from build123d import *

# Parameters (mm, degrees)
RESSALTO_EXTRUS_O1_DEPTH             = 52.5
ESBO_O3_W                            = 10
ESBO_O3_H                            = 4
RESSALTO_EXTRUS_O2_DEPTH             = 5
ESBO_O4_R                            = 1.7
ESBO_O4_W                            = 2.5
ESBO_O4_H                            = 5.6
RESSALTO_EXTRUS_O3_DEPTH             = 10
ESBO_O5_R                            = 1.65
CORTE_EXTRUS_O1_DEPTH                = 6
RESSALTO_EXTRUS_O4_REACH             = 12.6
ESBO_O6_W                            = 10
ESBO_O6_H                            = 2
RESSALTO_EXTRUS_O4_DIRECTION_2_REACH = 117.6


with BuildPart() as part:
    # Esboço1 → Ressalto-extrusão1 (new body, symmetric)
    with BuildSketch(Plane.XY):
        Polygon((0, 0), (0, 2), (5, 2), (5, 4), (10, 4), (10, 2), (20, 2), (20, 0), align=None)
    extrude(amount=RESSALTO_EXTRUS_O1_DEPTH, both=True)

    # Esboço3 → Ressalto-extrusão2 (add)
    with BuildSketch(Plane.XY.offset(52.5)):
        with Locations((5, 2)):
            Rectangle(ESBO_O3_W, ESBO_O3_H)
    extrude(amount=-RESSALTO_EXTRUS_O2_DEPTH)

    # Esboço4 → Ressalto-extrusão3 (add, through all)
    with BuildSketch(Plane(origin=(10, 0, 0), x_dir=(0, 0, -1), z_dir=(1, 0, 0))):
        Polygon((-52.5, 9.5), (-63.1, 9.5), (-63.1, 0), (-52.5, 0), (-52.5, 3.742943079), align=None)
        with Locations((-56.7, 4.7)):
            Circle(ESBO_O4_R, mode=Mode.SUBTRACT)
        with Locations((-59.85, 4.7)):
            Rectangle(ESBO_O4_W, ESBO_O4_H, mode=Mode.SUBTRACT)
    ressalto_extrus_o3 = extrude(amount=-RESSALTO_EXTRUS_O3_DEPTH)

    # Esboço5 → Corte-extrusão1 (cut)
    with BuildSketch(Plane.XY.offset(63.1)):
        with Locations((4, 4.7)):
            Circle(ESBO_O5_R)
    corte_extrus_o1 = extrude(amount=-CORTE_EXTRUS_O1_DEPTH, mode=Mode.SUBTRACT)

    # Espelhar1: Ressalto-extrusão3, Corte-extrusão1 across plane
    add(ressalto_extrus_o3.mirror(Plane.XY))
    add(corte_extrus_o1.mirror(Plane.XY), mode=Mode.SUBTRACT)

    # Ressalto-extrusão4: up to this face of the body (flat: up to its plane)
    ressalto_extrus_o4_end = Plane(part.part.faces().sort_by_distance((5, 9.362068858, 63.1))[0])
    # Esboço6 → Ressalto-extrusão4 (add, up to the picked face)
    with BuildSketch(Plane.XY.offset(52.5), mode=Mode.PRIVATE) as ressalto_extrus_o4_sk1:
        with Locations((15, 1)):
            Rectangle(ESBO_O6_W, ESBO_O6_H)
    ressalto_extrus_o4_tool1 = split(extrude(ressalto_extrus_o4_sk1.sketch, amount=RESSALTO_EXTRUS_O4_REACH, mode=Mode.PRIVATE), bisect_by=ressalto_extrus_o4_end, keep=Keep.BOTH, mode=Mode.PRIVATE)
    add(ressalto_extrus_o4_tool1.solids().sort_by_distance((15, 1, 52.5))[0])

    # Ressalto-extrusão4 direction 2: up to this face of the body (flat: up to its plane)
    ressalto_extrus_o4_direction_2_end = Plane(part.part.faces().sort_by_distance((5, 9.362068858, -63.1))[0])
    # Esboço6 → Ressalto-extrusão4 direction 2 (add, up to the picked face)
    with BuildSketch(Plane.XY.offset(52.5), mode=Mode.PRIVATE) as ressalto_extrus_o4_direction_2_sk1:
        with Locations((15, 1)):
            Rectangle(ESBO_O6_W, ESBO_O6_H)
    ressalto_extrus_o4_direction_2_tool1 = split(extrude(ressalto_extrus_o4_direction_2_sk1.sketch, amount=-RESSALTO_EXTRUS_O4_DIRECTION_2_REACH, mode=Mode.PRIVATE), bisect_by=ressalto_extrus_o4_direction_2_end, keep=Keep.BOTH, mode=Mode.PRIVATE)
    add(ressalto_extrus_o4_direction_2_tool1.solids().sort_by_distance((15, 1, 52.5))[0])


solid = part.part
Could you check a few things on this model? Use its own coordinates, in mm. A direction names the side the tool comes from. Give positions to 0.01 mm unless a question says otherwise; leave off trailing zeros. Order: outer loops, then holes, each group sorted by start corner. A loop starts at its lowest first (then second) coordinate and runs counter-clockwise, first axis right, second up.
Item 1: If we section it at A-A, the plane z = 7.5: Write out the boundary of the cut face in (x, y), plus the area to 3 significant figures.
Item 2: I need wall thicknesses on line 1 (X direction, y = 4.7, z = -62.45); line 2 (Y direction, x = 6.75, z = -56.7); line 3 (Z direction, x = 4.25, y = 4.7). Which ranges of each line are inside material? Lowest first, please.
Item 3: I'm going to push flat-ended pins straight in: pin 1 (11 mm diameter, centred on x = 4, z = 14.5, fed in from +Y); pin 2 (0.6 mm diameter, centred on y = 3, z = -9.5, fed in from -X); pin 3 (2 mm diameter, centred on x = 14.5, z = 6.5, fed in from +Y). Where does each tip first touch, or does it pass through?
Item 4: If we section it at B-B, the plane x = 17.5: Write out the boundary of the cut face in (y, z), plus the area to 3 significant figures.
Item 5: For faces 5 (the face through (5, 7, 52.5)), 6 (the face through (5, 3, -2)), 7 (the face through (5, 7.5, -60)), 8 (the face through (3.785, 6.336, 62.114)), which set-ups out of +Z, -Z, +X, -X, +Y, -Y let a thin tool reach every point of the face, with its end or its side?
Item 6: If we section it at C-C, the plane z = 51: Write out the boundary of the cut face in (x, y).
Item 7: If we mould it in two halves opening along X, with no side actions, what happens to faces 1 (the face through (4.89, 6.09, 58.03)), 2 (the face through (5, 9.5, 58)), 3 (the face through (0, 1.6, -0.3)), 4 (the face through (4.89, 6.09, -58.03))? For each: pulls with the +X half, pulls with the -X half, needs draft (parallel to the pull), parting line crosses it, or undercut.
Values:
1. outline: (0, 0) - (20, 0) - (20, 2) - (10, 2) - (10, 4) - (5, 4) - (5, 2) - (0, 2) - close
1. area: 50.0 mm2
2. line 1: x = 0 to 2.35, 5.65 to 10
2. line 2: y = 0 to 3, 6.4 to 9.5
2. line 3: z = -55 to -52.5, 52.5 to 55
3. pin 1: stops at y = 4
3. pin 2: stops at x = 5
3. pin 3: stops at y = 2
4. outline: (0, -63.1) - (2, -63.1) - (2, 63.1) - (0, 63.1) - close
4. area: 252 mm2
5. face 5: +X, -X, +Y
5. face 6: -X, +Y
5. face 7: +X, -X
5. face 8: +Z
6. outline: (0, 0) - (20, 0) - (20, 2) - (10, 2) - (10, 4) - (0, 4) - close
7. face 1: undercut
7. face 2: needs draft
7. face 3: pulls with the -X half
7. face 4: undercut
